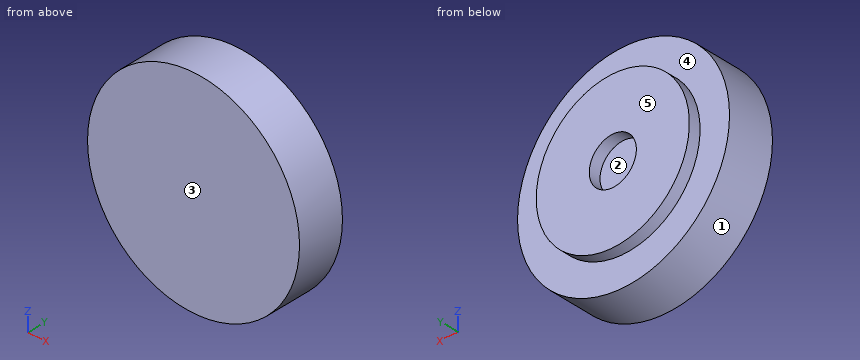
```python
from build123d import *

# Parameters (mm, degrees)
SKETCH_1_R          = 9
EXTRUDE_1_DEPTH     = 5
SKETCH_2_OUTSIDE_W  = 25.188
SKETCH_2_OUTSIDE_H  = 25.188
SKETCH_2_OUTSIDE_R  = 6.5
CUT_EXTRUDE_1_DEPTH = 1
SKETCH_3_R          = 2
CUT_EXTRUDE_2_DEPTH = 1


with BuildPart() as part:
    # 草图1 → 凸台-拉伸1 (new body)
    with BuildSketch(Plane(origin=(0, 0, 0), x_dir=(1, 0, 0), z_dir=(0, 1, 0))):
        Circle(SKETCH_1_R)
    extrude(amount=EXTRUDE_1_DEPTH)

    # 草图2 outside → 切除-拉伸1 (cut)
    with BuildSketch(Plane(origin=(0, 5, 0), x_dir=(1, 0, 0), z_dir=(0, 1, 0))):
        Rectangle(SKETCH_2_OUTSIDE_W, SKETCH_2_OUTSIDE_H)
        Circle(SKETCH_2_OUTSIDE_R, mode=Mode.SUBTRACT)
    extrude(amount=-CUT_EXTRUDE_1_DEPTH, mode=Mode.SUBTRACT)

    # 草图3 → 切除-拉伸2 (cut)
    with BuildSketch(Plane(origin=(0, 5, 0), x_dir=(1, 0, 0), z_dir=(0, 1, 0))):
        Circle(SKETCH_3_R)
    extrude(amount=-CUT_EXTRUDE_2_DEPTH, mode=Mode.SUBTRACT)


solid = part.part
```
Geometry: final body of the model. Coordinates: model frame, mm. Face numbers are marked on the shaded views. A direction names the side the tool comes from. Round coordinates to 2 decimals unless told otherwise and drop trailing zeros. Loops run counter-clockwise (first coordinate to the right, second up) from the corner with the lowest first, then second, coordinate; pieces in that order, holes last. Notation, with made-up numbers: (27, -37) -> (82, -37) arc R5 cw to (82, -33) -> close; hole circle Ø5 at (-38.75, 47). An arc over 180 degrees is marked (long way). Use one line per item in the form item = value. Start each with the question number.
1) Section D-D on z = 4. Output: boundary loops of the cut face in (x, y).
2) Draft query along Z for the marked faces 1, 2 and 3. Return one class per face: released by +Z, released by -Z, zero draft, split by the parting line, or undercut.
3) Line query: L1, parallel to X at y = 4.3, z = 0; L2, parallel to Y at x = 7, z = -4.75. Output: solid intervals per line, ascending.
4) Section A-A on x = 0. Output: boundary loops of the cut face in (y, z), then the cut area to 3 significant figures.
5) First-contact query: P1, Ø2, axis at x = 0, z = 0, coming from the +Y side; P2, Ø1, axis at y = 1.5, z = 3, coming from the -X side; P3, Ø1.5, axis at y = 1, z = 4.5, coming from the -X side. Flat tips, straight axial feed; report the tip coordinate or a pass-through.
6) Section C-C on y = 3.2. Output: boundary loops of the cut face in (x, z), then the cut area to 3 significant figures.
7) Access query for the marked faces 4 and 5. Directions: +Z, -Z, +X, -X, +Y, -Y. A direction counts if a zero-diameter tool reaches every point of the face in a straight line with its end or side. Return the directions, or none.
8) Section B-B on z = 0. Output: boundary loops of the cut face in (x, y).
Response:
q1.outline = (-8.06, 0) -> (8.06, 0) -> (8.06, 4) -> (5.12, 4) -> (5.12, 5) -> (-5.12, 5) -> (-5.12, 4) -> (-8.06, 4) -> close
q2.face_1 = split by the parting line
q2.face_2 = undercut
q2.face_3 = zero draft
q3.L1 = -6.5 to -2, 2 to 6.5
q3.L2 = 0 to 4
q4.outline = (0, -9) -> (4, -9) -> (4, -6.5) -> (5, -6.5) -> (5, -2) -> (4, -2) -> (4, 2) -> (5, 2) -> (5, 6.5) -> (4, 6.5) -> (4, 9) -> (0, 9) -> close
q4.area = 81.0 mm^2
q5.P1 = 4
q5.P2 = -8.65
q5.P3 = -8.18
q6.outline = circle Ø18 at (0, 0)
q6.area = 254 mm^2
q7.face_4 = +Y
q7.face_5 = +Z, -Z, +X, -X, +Y
q8.outline = (-9, 0) -> (9, 0) -> (9, 4) -> (6.5, 4) -> (6.5, 5) -> (2, 5) -> (2, 4) -> (-2, 4) -> (-2, 5) -> (-6.5, 5) -> (-6.5, 4) -> (-9, 4) -> close
